Check sheet for the drawn part. Datum: minimum x, y, z corner. Units: mm. Give positions to 0.01 mm unless a question says otherwise; leave off trailing zeros. Write each loop counter-clockwise with the first axis right and the second up, starting at its lowest first coordinate (ties: lowest second). Pieces come first, ordered by that corner, then holes.
(1) Cross-section at B-B (x = 209). Record the boundary of the cut face in (y, z).
(2) Cross-section at C-C (x = 133). Record the boundary of the cut face in (y, z).
(3) Depth check by flat-ended pin: P1, Ø9, axis at y = 32, z = 211.5, coming from the +X side; P2, Ø11, axis at x = 109.5, y = 19.5, coming from the -Z side; P3, Ø20, axis at y = 32.5, z = 218.5, coming from the -X side; P4, Ø7, axis at y = 35, z = 215, coming from the -X side. Enter the tip coordinate at first touch or a pass-through.
(4) Thickness scan on line 1 along Y through (x, z) = (112, 215); line 2 along Z through (x, y) = (137, 7.5); line 3 along Z through (x, y) = (66.5, 21). Record the ranges inside material, lowest first.
(5) Cross-section at A-A (y = 21). Record the boundary of the cut face in (x, z), and give its area (3 significant figures).
(6) Cross-section at D-D (z = 215). Count the separate pieces of the cut face and the enclosed holes in it, and give its area (3 significant figures).
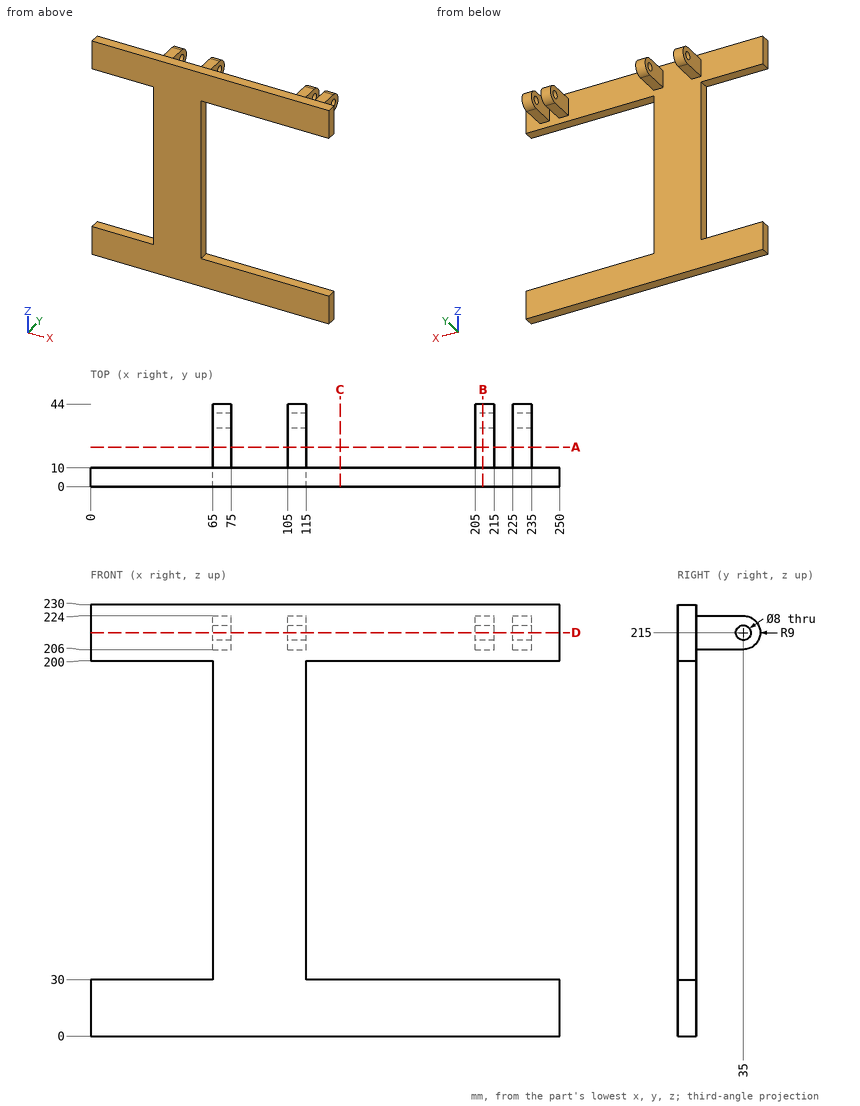
Reply:
1. outline: (0, 0) - (10, 0) - (10, 30) - (0, 30) - close; (0, 200) - (10, 200) - (10, 206) - (35, 206) arc R9 ccw to (35, 224) - (10, 224) - (10, 230) - (0, 230) - close; hole circle Ø8 at (35, 215)
2. outline: (0, 0) - (10, 0) - (10, 30) - (0, 30) - close; (0, 200) - (10, 200) - (10, 230) - (0, 230) - close
3. P1: stops at x = 235
3. P2: stops at z = 206
3. P3: stops at x = 65
3. P4: passes through
4. line 1: y = 0 to 31, 39 to 44
4. line 2: z = 0 to 30, 200 to 230
4. line 3: z = 206 to 224
5. outline: (65, 206) - (75, 206) - (75, 224) - (65, 224) - close; (105, 206) - (115, 206) - (115, 224) - (105, 224) - close; (205, 206) - (215, 206) - (215, 224) - (205, 224) - close; (225, 206) - (235, 206) - (235, 224) - (225, 224) - close
5. area: 720 mm2
6. separate pieces: 5
6. enclosed holes: 0
6. area: 3,540 mm2
